Part model, mm, in its own coordinate system. Give positions to 0.01 mm unless a question says otherwise; leave off trailing zeros. Order: outer loops, then holes, each group sorted by start corner. A loop starts at its lowest first (then second) coordinate and runs counter-clockwise, first axis right, second up. Notation, with made-up numbers: (-19.75, 65) - (-6.75, 65) arc R11 cw to (-6.75, 73) - close; hole circle Ø2 at (88.5, 82.5). An arc over 180 degrees is marked (long way). One line per item, written item: value.
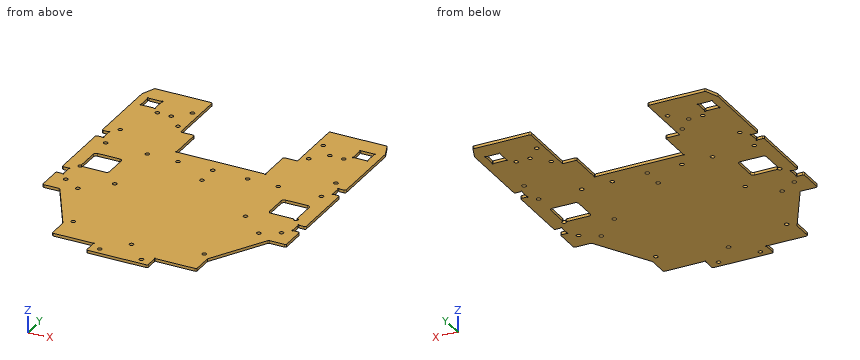
```python
from build123d import *

# Parameters (mm, degrees)
SKETCH_1_R          = 1.5
SKETCH_1_W          = 10.2
SKETCH_1_H          = 10.2
EXTRUDE_3_DEPTH     = 2
SKETCH_3_R          = 1.5
SKETCH_3_W          = 5.1
SKETCH_3_H          = 8.2
CUT_EXTRUDE_2_DEPTH = 3
SKETCH_4_W          = 10
SKETCH_4_H          = 25
EXTRUDE_4_DEPTH     = 2
SKETCH_2_R          = 0.5
CUT_EXTRUDE_1_DEPTH = 3
FILLET_1_R          = 1
CUT_EXTRUDE_3_DEPTH = 10
SKETCH_6_R          = 1.5
CUT_EXTRUDE_4_DEPTH = 10


with BuildPart() as part:
    # 草图1 → 凸台-拉伸3 (new body)
    with BuildSketch(Plane.XY):
        Polygon((-87.5, 69), (-87.5, -77.9), (-74.994010768, -77.9), (-51.9, -117.9), (-51.9, -132.9), (-22, -132.9), (-22, -143), (22, -143), (22, -132.9), (51.9, -132.9), (51.9, -117.9), (74.994010768, -77.9), (87.5, -77.9), (87.5, 69), (42, 69), (42, 0), (-42, 0), (-42, 69), align=None)
        with Locations((-25, -11)):
            Circle(SKETCH_1_R, mode=Mode.SUBTRACT)
        with Locations((0, -26)):
            Circle(SKETCH_1_R, mode=Mode.SUBTRACT)
        with Locations((-47, -11)):
            Circle(SKETCH_1_R, mode=Mode.SUBTRACT)
        with Locations((-15, -138)):
            Circle(SKETCH_1_R, mode=Mode.SUBTRACT)
        with Locations((0, -123)):
            Circle(SKETCH_1_R, mode=Mode.SUBTRACT)
        with Locations((47, -11)):
            Circle(SKETCH_1_R, mode=Mode.SUBTRACT)
        with Locations((25, -11)):
            Circle(SKETCH_1_R, mode=Mode.SUBTRACT)
        with Locations((15, -138)):
            Circle(SKETCH_1_R, mode=Mode.SUBTRACT)
        with Locations((0, -11)):
            Circle(SKETCH_1_R, mode=Mode.SUBTRACT)
        with Locations((-47, 51)):
            Circle(SKETCH_1_R, mode=Mode.SUBTRACT)
        with Locations((47, 51)):
            Circle(SKETCH_1_R, mode=Mode.SUBTRACT)
        with Locations((-47, -113)):
            Circle(SKETCH_1_R, mode=Mode.SUBTRACT)
        with Locations((-47, -56)):
            Circle(SKETCH_1_R, mode=Mode.SUBTRACT)
        with Locations((47, -56)):
            Circle(SKETCH_1_R, mode=Mode.SUBTRACT)
        with Locations((47, -113)):
            Circle(SKETCH_1_R, mode=Mode.SUBTRACT)
        with Locations((-47, 31)):
            Circle(SKETCH_1_R, mode=Mode.SUBTRACT)
        with Locations((-67, 41)):
            Circle(SKETCH_1_R, mode=Mode.SUBTRACT)
        with Locations((-57, 41)):
            Circle(SKETCH_1_R, mode=Mode.SUBTRACT)
        with Locations((57, 41)):
            Circle(SKETCH_1_R, mode=Mode.SUBTRACT)
        with Locations((67, 41)):
            Circle(SKETCH_1_R, mode=Mode.SUBTRACT)
        with Locations((47, 31)):
            Circle(SKETCH_1_R, mode=Mode.SUBTRACT)
        with Locations((76.3, 50.7)):
            Rectangle(SKETCH_1_W, SKETCH_1_H, mode=Mode.SUBTRACT)
        with Locations((-76.3, 50.7)):
            Rectangle(SKETCH_1_W, SKETCH_1_H, mode=Mode.SUBTRACT)
    extrude(amount=EXTRUDE_3_DEPTH)

    # 草图3 → 切除-拉伸2 (cut, through all)
    with BuildSketch(Plane.XY.offset(2)):
        with Locations((77.5, 10)):
            Circle(SKETCH_3_R)
        with Locations((77.5, -10)):
            Circle(SKETCH_3_R)
        with Locations((77.5, -45)):
            Circle(SKETCH_3_R)
        with Locations((77.5, -65)):
            Circle(SKETCH_3_R)
        with Locations((-77.5, -45)):
            Circle(SKETCH_3_R)
        with Locations((-77.5, -65)):
            Circle(SKETCH_3_R)
        with Locations((-77.5, -10)):
            Circle(SKETCH_3_R)
        with Locations((-77.5, 10)):
            Circle(SKETCH_3_R)
        with Locations((84.95, 0)):
            Rectangle(SKETCH_3_W, SKETCH_3_H)
        with Locations((-84.95, 0)):
            Rectangle(SKETCH_3_W, SKETCH_3_H)
        with Locations((-84.95, -55)):
            Rectangle(SKETCH_3_W, SKETCH_3_H)
        with Locations((84.95, -55)):
            Rectangle(SKETCH_3_W, SKETCH_3_H)
        Polygon((83.459737742, 69), (87.5, 59), (87.5, 69), align=None)
        Polygon((-87.5, 59), (-87.5, 69), (-83.459737742, 69), align=None)
    extrude(amount=-CUT_EXTRUDE_2_DEPTH, mode=Mode.SUBTRACT)

    # 草图4 → 凸台-拉伸4 (add)
    with BuildSketch(Plane(origin=(0, 0, 0), x_dir=(-1, 0, 0), z_dir=(0, 0, -1))):
        with Locations((-37, 12.5)):
            Rectangle(SKETCH_4_W, SKETCH_4_H)
        with Locations((37, 12.5)):
            Rectangle(SKETCH_4_W, SKETCH_4_H)
    extrude(amount=-EXTRUDE_4_DEPTH)

    # 草图2 → 切除-拉伸1 (cut, through all)
    with BuildSketch(Plane.XY.offset(2)):
        with Locations((-81.4, 45.6)):
            Circle(SKETCH_2_R)
        with Locations((-81.4, 55.8)):
            Circle(SKETCH_2_R)
        with Locations((-71.2, 45.6)):
            Circle(SKETCH_2_R)
        with Locations((-71.2, 55.8)):
            Circle(SKETCH_2_R)
        with Locations((71.2, 55.8)):
            Circle(SKETCH_2_R)
        with Locations((71.2, 45.6)):
            Circle(SKETCH_2_R)
        with Locations((81.4, 55.8)):
            Circle(SKETCH_2_R)
        with Locations((81.4, 45.6)):
            Circle(SKETCH_2_R)
        with Locations((82.4, 4.1)):
            Circle(SKETCH_2_R)
        with Locations((82.4, -4.1)):
            Circle(SKETCH_2_R)
        with Locations((82.4, -50.9)):
            Circle(SKETCH_2_R)
        with Locations((82.4, -59.1)):
            Circle(SKETCH_2_R)
        with Locations((22, -132.9)):
            Circle(SKETCH_2_R)
        with Locations((-82.4, -59.1)):
            Circle(SKETCH_2_R)
        with Locations((-82.4, -50.9)):
            Circle(SKETCH_2_R)
        with Locations((-82.4, -4.1)):
            Circle(SKETCH_2_R)
        with Locations((-82.4, 4.1)):
            Circle(SKETCH_2_R)
        with Locations((-22, -132.9)):
            Circle(SKETCH_2_R)
        with Locations((32, 0)):
            Circle(SKETCH_2_R)
        with Locations((-32, 0)):
            Circle(SKETCH_2_R)
    extrude(amount=-CUT_EXTRUDE_1_DEPTH, mode=Mode.SUBTRACT)

    # 圆角1
    fillet_1_edges = [part.edges().sort_by_distance(p)[0] for p in [
        (87.5, -50.9, 1),
        (87.5, -59.1, 1),
        (-87.5, -59.1, 1),
        (-87.5, -50.9, 1),
        (-87.5, -4.1, 1),
        (-87.5, 4.1, 1),
        (83.459737742, 69, 1),
        (87.5, 59, 1),
        (-83.459737742, 69, 1),
        (-87.5, 59, 1),
        (87.5, 4.1, 1),
        (87.5, -4.1, 1),
        (32, 25, 1),
        (-32, 25, 1),
        (-87.5, -77.9, 1),
        (-42, 69, 1),
        (42, 69, 1),
        (87.5, -77.9, 1),
        (74.994010768, -77.9, 1),
        (51.9, -132.9, 1),
        (22, -143, 1),
        (-22, -143, 1),
        (-51.9, -132.9, 1),
        (-74.994010768, -77.9, 1),
    ]]
    fillet(fillet_1_edges, radius=FILLET_1_R)

    # 草图5 → 切除-拉伸3 (cut)
    with BuildSketch(Plane.XY.offset(2)):
        with BuildLine():
            Line((-75.5, -25), (-59.5, -25))
            ThreePointArc((-59.5, -25), (-58.085786438, -25.585786438), (-57.5, -27))
            Line((-57.5, -27), (-57.5, -43))
            ThreePointArc((-57.5, -43), (-58.085786438, -44.414213562), (-59.5, -45))
            Line((-59.5, -45), (-75.5, -45))
            ThreePointArc((-75.5, -45), (-76.914213562, -44.414213562), (-77.5, -43))
            Line((-77.5, -43), (-77.5, -27))
            ThreePointArc((-77.5, -27), (-76.914213562, -25.585786438), (-75.5, -25))
        make_face()
        with BuildLine():
            Line((75.5, -45), (59.5, -45))
            ThreePointArc((59.5, -45), (58.085786438, -44.414213562), (57.5, -43))
            Line((57.5, -43), (57.5, -27))
            ThreePointArc((57.5, -27), (58.085786438, -25.585786438), (59.5, -25))
            Line((59.5, -25), (75.5, -25))
            ThreePointArc((75.5, -25), (76.914213562, -25.585786438), (77.5, -27))
            Line((77.5, -27), (77.5, -43))
            ThreePointArc((77.5, -43), (76.914213562, -44.414213562), (75.5, -45))
        make_face()
    extrude(amount=-CUT_EXTRUDE_3_DEPTH, mode=Mode.SUBTRACT)

    # 草图6 → 切除-拉伸4 (cut)
    with BuildSketch(Plane.XY.offset(2)):
        with Locations((-65, -72.2)):
            Circle(SKETCH_6_R)
        with Locations((65, -72.2)):
            Circle(SKETCH_6_R)
    extrude(amount=-CUT_EXTRUDE_4_DEPTH, mode=Mode.SUBTRACT)


solid = part.part
```
1) Cut at B-B, the plane z = 1.35. Give the number of separate pieces and of enclosed holes in the cut face, then the cut area to 3 significant figures.
Outcome:
separate pieces: 1
enclosed holes: 33
area: 26,000 mm^2
2) Cut at C-C, the plane x = 11. Give the cut face in (y, z), then the cut area to 3 significant figures.
Outcome:
outline: (-143, 0) - (0, 0) - (0, 2) - (-143, 2) - close
area: 286 mm^2
3) Cut at A-A, the plane y = 36. Give the cut face in (x, z), then the cut area to 3 significant figures.
Outcome:
outline: (-87.5, 0) - (-42, 0) - (-42, 2) - (-87.5, 2) - close; (42, 0) - (87.5, 0) - (87.5, 2) - (42, 2) - close
area: 182 mm^2
4) Drill centre lines: line 1 along X through (y, z) = (-35.5, 0.8); line 2 along Y through (x, z) = (47, 0.55); line 3 along Y through (x, z) = (0, 1.2). Where is each one in solid material? Low to high. Write a range as from..to.
Outcome:
line 1: x = -87.5..-77.5, -57.5..57.5, 77.5..87.5
line 2: y = -132.9..-114.5, -111.5..-57.5, -54.5..-12.5, -9.5..29.5, 32.5..49.5, 52.5..69
line 3: y = -143..-124.5, -121.5..-27.5, -24.5..-12.5, -9.5..0
5) Cut at D-D, the plane y = -97.5. Give the cut face in (x, z), then the cut area to 3 significant figures.
Outcome:
outline: (-63.68, 0) - (63.68, 0) - (63.68, 2) - (-63.68, 2) - close
area: 255 mm^2
6) Pin check, flat tips, straight feed: pin 1 (3.5 mm diameter, centred on x = -77.5, y = -10, fed in from +Z); pin 2 (2.5 mm diameter, centred on x = 47, y = 31, fed in from +Z); pin 3 (1 mm diameter, centred on y = -2, z = 0.5, fed in from -X). Stop position of each tip, or through.
Outcome:
pin 1: stops at z = 2
pin 2: passes through
pin 3: stops at x = -82.4
